Can you work these out from the model? Positions are in its coordinate system, mm. A direction names the side the tool comes from. Give positions to 0.01 mm unless a question says otherwise; leave off trailing zeros. Write each loop counter-clockwise with the first axis right and the second up, starting at its lowest first coordinate (ties: lowest second). Pieces come first, ordered by that corner, then holes.
```python
from build123d import *

# Parameters (mm, degrees)
SKETCH_1_W               = 105
SKETCH_1_H               = 125
EXTRUDE_1_DEPTH          = 115
CUT_EXTRUDE_1_DEPTH      = 1
CUT_EXTRUDE_1_DEPTH_BACK = 126


with BuildPart() as part:
    # Эскиз1 → Бобышка-Вытянуть1 (new body)
    with BuildSketch(Plane(origin=(0, 0, 0), x_dir=(1, 0, 0), z_dir=(0, 1, 0))):
        Rectangle(SKETCH_1_W, SKETCH_1_H)
    extrude(amount=EXTRUDE_1_DEPTH)

    # Эскиз2 → Вырез-Вытянуть1 (cut, two sides)
    with BuildSketch(Plane.XY.offset(62.5)) as cut_extrude_1_sk:
        with BuildLine():
            ThreePointArc((-52.5, 62.5), (-46.071684117, 87.67240399), (-28.360955327, 106.680382671))
            Line((-28.360955327, 106.680382671), (-28.360955327, 115))
            Line((-28.360955327, 115), (-52.5, 115))
            Line((-52.5, 115), (-52.5, 62.5))
        make_face()
        with BuildLine():
            ThreePointArc((-31.408561264, 20.43157622), (-46.931862665, 38.970225951), (-52.5, 62.5))
            Line((-52.5, 62.5), (-52.5, 20.43157622))
            Line((-52.5, 20.43157622), (-31.408561264, 20.43157622))
        make_face()
        with BuildLine():
            Line((52.5, 20.43157622), (52.5, 62.499999878))
            ThreePointArc((52.5, 62.499999878), (46.931862637, 38.970225896), (31.408561264, 20.43157622))
            Line((31.408561264, 20.43157622), (52.5, 20.43157622))
        make_face()
        with BuildLine():
            Line((52.5, 115), (28.360955327, 115))
            Line((28.360955327, 115), (28.360955327, 106.680382671))
            ThreePointArc((28.360955327, 106.680382671), (46.071684146, 87.672403937), (52.5, 62.499999878))
            Line((52.5, 62.499999878), (52.5, 115))
        make_face()
    extrude(amount=CUT_EXTRUDE_1_DEPTH, mode=Mode.SUBTRACT)
    extrude(cut_extrude_1_sk.sketch, amount=-CUT_EXTRUDE_1_DEPTH_BACK, mode=Mode.SUBTRACT)


solid = part.part
```
1) For pin 1 Ø8 at (y, z) = (51.5, 36.5) entering from +X; pin 2 Ø10 at (y, z) = (96.5, 34) entering from -X; pin 3 Ø8 at (x, z) = (-41.5, 29) entering from +Y, each with a flat end and sliding along its axis, tell me the tip position at first contact or that it passes through.
Values follow:
pin 1: stops at x = 52.03
pin 2: stops at x = -43.76
pin 3: stops at y = 99.24
2) For faces 4 (the face through (28.361, 111, 1)), 5 (the face through (52.5, 10, 1)), 6 (the face through (-28.361, 111, 1)), which set-ups out of +Z, -Z, +X, -X, +Y, -Y let a thin tool reach every point of the face, with its end or its side?
Values follow:
face 4: +Z, -Z, +X, +Y
face 5: +Z, -Z, +X, +Y, -Y
face 6: +Z, -Z, -X, +Y
3) Suppose I cut it at A-A on z = 49.5. Write out the boundary of the cut face in (x, y).
Values follow:
outline: (-52.5, 0) - (52.5, 0) - (52.5, 20.43) - (31.41, 20.43) arc R52.5 ccw to (28.36, 106.68) - (28.36, 115) - (-28.36, 115) - (-28.36, 106.68) arc R52.5 ccw to (-31.41, 20.43) - (-52.5, 20.43) - close
4) Suppose I cut it at C-C on y = 33.5. Write out the boundary of the cut face in (x, z).
Values follow:
outline: (-43.76, -62.5) - (43.76, -62.5) - (43.76, 62.5) - (-43.76, 62.5) - close
5) Please list where these lines run through material, in increasing order: L1, parallel to Y at x = -40, z = 28.5; L2, parallel to Y at x = 43.5, z = -31; L3, parallel to X at y = 61.5, z = -9.5.
Values follow:
L1: y = 0 to 20.43, 28.5 to 96.5
L2: y = 0 to 20.43, 33.11 to 91.89
L3: x = -52.49 to 52.49
6) Suppose I cut it at B-B on y = 94. Write out the boundary of the cut face in (x, z), plus the area to 3 significant figures.
Values follow:
outline: (-42, -62.5) - (42, -62.5) - (42, 62.5) - (-42, 62.5) - close
area: 10,500 mm2
7) If we mould it in two halves opening along Y, with no side actions, what happens to faces 1 (the face through (-1, 57, 62.5)), 2 (the face through (0, 115, -1)), 3 (the face through (-42, 20.432, 1))? For each: +Y half, -Y half, draft (parallel to the pull), parting line (faces both ways), or undercut.
Values follow:
face 1: draft
face 2: +Y half
face 3: undercut
